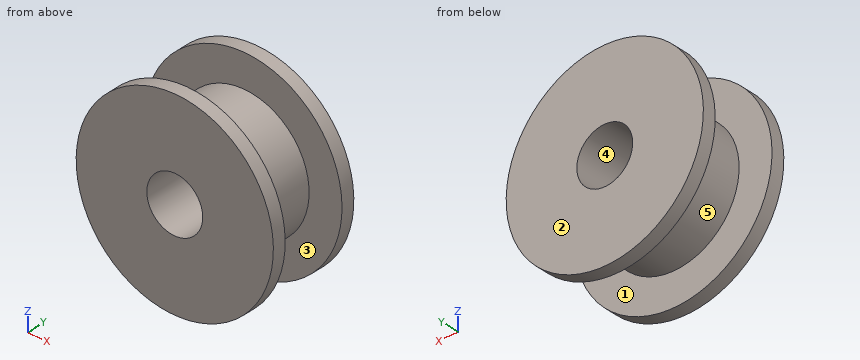
from build123d import *

# Parameters (mm, degrees)
SKETCH_1_R          = 6
EXTRUDE_1_DEPTH     = 3
SKETCH_3_R          = 9
EXTRUDE_2_DEPTH     = 1.25
SKETCH_4_R          = 2.55
CUT_EXTRUDE_1_DEPTH = 16.305227865


with BuildPart() as part:
    # 草图1 → 凸台-拉伸1 (new, symmetric)
    with BuildSketch(Plane(origin=(0, 0, 0), x_dir=(1, 0, 0), z_dir=(0, 1, 0))):
        with Locations(Location((0, 0, 0), (0, 0, 270))):
            Circle(SKETCH_1_R)
    extrude(amount=EXTRUDE_1_DEPTH, both=True)

    # 草图3 → 凸台-拉伸2 (add)
    with BuildSketch(Plane(origin=(0, 3, 0), x_dir=(1, 0, 0), z_dir=(0, 1, 0))):
        with Locations(Location((0, 0, 0), (0, 0, 270))):
            Circle(SKETCH_3_R)
    extrude_2 = extrude(amount=EXTRUDE_2_DEPTH)

    # 镜向1: 凸台-拉伸2 across plane
    add(extrude_2.mirror(Plane.ZX))

    # 草图4 → 切除-拉伸1 (cut, through all)
    with BuildSketch(Plane(origin=(0, 4.25, 0), x_dir=(1, 0, 0), z_dir=(0, 1, 0))):
        with Locations(Location((0, 0, 0), (0, 0, 270))):
            Circle(SKETCH_4_R)
    extrude(amount=-CUT_EXTRUDE_1_DEPTH, mode=Mode.SUBTRACT)


solid = part.part
Input: part model. Units: mm. Frame: model coordinates. Face numbers are marked on the shaded views. A direction names the side the tool comes from. Give positions to 0.01 mm unless a question says otherwise; leave off trailing zeros. Loops run counter-clockwise (first coordinate to the right, second up) from the corner with the lowest first, then second, coordinate; pieces in that order, holes last. Notation, with made-up numbers: M 84.25,-33 L 97.25,-33 A28 cw 97.25,-5 Z; hole C 9,-20.75 d4. An arc over 180 degrees is marked long. Use one line per item in the form item = value.
1. Pull-direction query (X, two-part tool) for the marked faces 3, 4 and 5; classes: released by +X, released by -X, zero draft, split by the parting line, or undercut.
Numbers:
face_3 = zero draft
face_4 = undercut
face_5 = split by the parting line
2. Section query D-D, the plane x = -4.5. Return the cut outline in (y, z).
Numbers:
outline = M -4.25,-7.79 L -3,-7.79 L -3,-3.97 L 3,-3.97 L 3,-7.79 L 4.25,-7.79 L 4.25,7.79 L 3,7.79 L 3,3.97 L -3,3.97 L -3,7.79 L -4.25,7.79 Z
3. Section query B-B, the plane z = 7. Return the cut outline in (x, y), and give its area (3 significant figures).
Numbers:
outline = M -5.66,-4.25 L 5.66,-4.25 L 5.66,-3 L -5.66,-3 Z; M -5.66,3 L 5.66,3 L 5.66,4.25 L -5.66,4.25 Z
area = 28.3 mm²
4. Section query C-C, the plane y = 1.25. Return the cut outline in (x, z).
Numbers:
outline = C 0,0 d12; hole C 0,0 d5.1
5. Reachability of the marked faces 1 and 2 from +Z, -Z, +X, -X, +Y, -Y: full face, straight path, thin tool, end or side. Return the list, or none.
Numbers:
face_1 = none
face_2 = +Z, -Z, +X, -X, +Y
6. Section query A-A, the plane x = 0. Return the cut outline in (y, z).
Numbers:
outline = M -4.25,-9 L -3,-9 L -3,-6 L 3,-6 L 3,-9 L 4.25,-9 L 4.25,-2.55 L -4.25,-2.55 Z; M -4.25,2.55 L 4.25,2.55 L 4.25,9 L 3,9 L 3,6 L -3,6 L -3,9 L -4.25,9 Z
7. First-contact query: pin 1 (4.5 mm diameter, centred on x = 0, z = 0, fed in from -Y); pin 2 (5 mm diameter, centred on x = 3.5, y = -2, fed in from +Z). Flat tips, straight axial feed; report the tip coordinate or a pass-through.
Numbers:
pin_1 = through
pin_2 = 8.92
8. Line query: L1, parallel to Y at x = -6.5, z = -5.25; L2, parallel to X at y = 1.25, z = 0; L3, parallel to X at y = 2.75, z = 1.5. Output: solid intervals per line, ascending.
Numbers:
L1 = -4.25 to -3, 3 to 4.25
L2 = -6 to -2.55, 2.55 to 6
L3 = -5.81 to -2.06, 2.06 to 5.81
